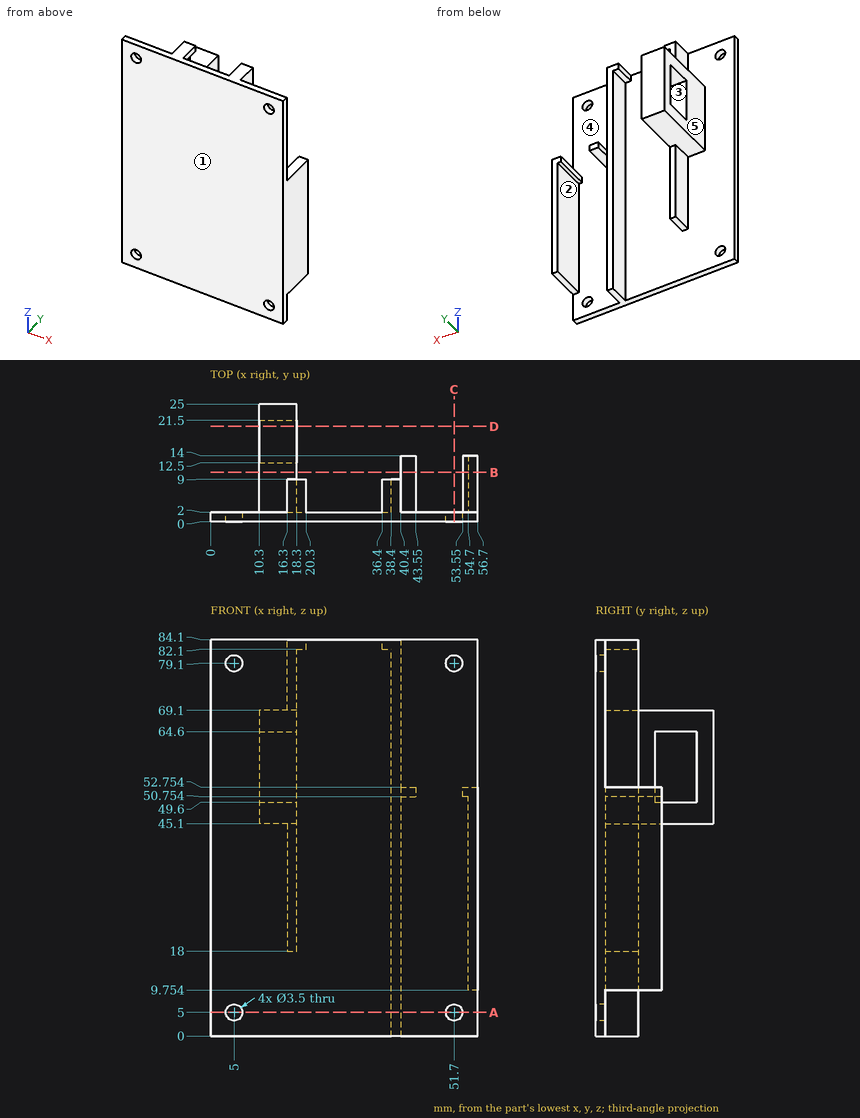
For this review, use the dimensioned drawing (mm, ordinates from the lowest corner) and the shaded views. A direction names the side the tool comes from. Coordinates: 2 decimals unless noted, no trailing zeros. Order: outer loops, then holes, each group sorted by start corner. A loop starts at its lowest first (then second) coordinate and runs counter-clockwise, first axis right, second up. Notation, with made-up numbers: (-25.75, -7) - (2.25, -7) arc R19 cw to (2.25, 30) - close; hole circle Ø6 at (-14, -10). An arc over 180 degrees is marked (long way). Use one line per item in the form item = value.
Q1. Consider section A-A (z = 5). Give the boundary of the cut face in (x, y), then the cut area to 3 significant figures.
Checked values:
outline = (0, 0) - (3.25, 0) - (3.25, 2) - (0, 2) - close; (6.75, 0) - (49.95, 0) - (49.95, 2) - (40.4, 2) - (40.4, 9) - (38.4, 9) - (38.4, 2) - (6.75, 2) - close; (53.45, 0) - (56.7, 0) - (56.7, 2) - (53.45, 2) - close
area = 113 mm2
Q2. For the marked faces 1 and 2, list the 3-axis set-ups (+Z, -Z, +X, -X, +Y, -Y) from which the entire face can be reached by the end or side of a thin tool; tool diameter is ignored.
Checked values:
face_1 = +Z, -Z, +X, -X, -Y
face_2 = -Z, +Y
Q3. Draft analysis for pull direction X (two halves, no side actions). For the marked faces 3, 4 and 5, state which applies: +X half, -X half, draft (parallel to the pull), parting line (faces both ways), or undercut.
Checked values:
face_3 = draft
face_4 = undercut
face_5 = -X half
Q4. For P1, Ø3, axis at y = 4, z = 36.5, coming from the -X side; P2, Ø1.6, axis at y = 8.5, z = 52, coming from the -X side; P3, Ø6.5, axis at x = 15.5, y = 15.5, coming from the -Z side, all flat-tipped, find the tip position at first contact; note any pin that passes through.
Checked values:
P1 = 16.3
P2 = 10.3
P3 = 45.1
Q5. Consider section B-B (y = 10.5). Give the boundary of the cut face in (x, z), then the cut area to 3 significant figures.
Checked values:
outline = (10.3, 45.1) - (18.3, 45.1) - (18.3, 69.1) - (10.3, 69.1) - close; (40.4, 50.75) - (43.55, 50.75) - (43.55, 52.75) - (40.4, 52.75) - close; (53.55, 50.75) - (54.7, 50.75) - (54.7, 9.75) - (56.7, 9.75) - (56.7, 52.75) - (53.55, 52.75) - close
area = 287 mm2
Q6. For probe 1 along Z at (x, y) = (51.7, 1.45); probe 2 along X at (y, z) = (7.75, 50); probe 3 along X at (y, z) = (1.1, 79.1), list the stretches that pass through material, from the lowest coordinate up. Write a range as from..to.
Checked values:
probe_1 = 0..3.25, 6.75..77.35, 80.85..84.1
probe_2 = 10.3..18.3, 38.4..40.4, 54.7..56.7
probe_3 = 0..3.25, 6.75..49.95, 53.45..56.7
Q7. Consider section D-D (y = 20.25). Give the boundary of the cut face in (x, z).
Checked values:
outline = (10.3, 45.1) - (18.3, 45.1) - (18.3, 49.6) - (10.3, 49.6) - close; (10.3, 64.6) - (18.3, 64.6) - (18.3, 69.1) - (10.3, 69.1) - close
Q8. Consider section C-C (x = 51.7). Give the boundary of the cut face in (y, z), then the cut area to 3 significant figures.
Checked values:
outline = (0, 0) - (2, 0) - (2, 3.25) - (0, 3.25) - close; (0, 6.75) - (2, 6.75) - (2, 77.35) - (0, 77.35) - close; (0, 80.85) - (2, 80.85) - (2, 84.1) - (0, 84.1) - close
area = 154 mm2
